```python
from build123d import *

# Parameters (mm, degrees)
SKETCH1_R           = 2.286
MAIN_BODY_DEPTH     = 1.5875
SKETCH2_R           = 2.286
MOUNT_HOLES_DEPTH   = 2.5875
SKETCH3_R           = 1.5875
OLD_PCB_HOLES_DEPTH = 2.54


with BuildPart() as part:
    # Sketch1 → Main Body (new body)
    with BuildSketch(Plane(origin=(0, 0, 0), x_dir=(1, 0, 0), z_dir=(0, 1, 0))):
        Polygon((-25.4, 86.995), (-63.43142, 86.995), (-63.43142, 60.96), (-78.74, 60.96), (-78.74, 25.4), (-71.12, 25.4), (-71.12, -25.4), (-78.74, -25.4), (-78.74, -60.96), (-63.43142, -60.96), (-63.43142, -86.995), (-25.4, -86.995), (-25.4, -79.375), (25.4, -79.375), (25.4, -86.995), (63.43142, -86.995), (63.43142, -60.96), (78.74, -60.96), (78.74, -25.4), (71.12, -25.4), (71.12, 25.4), (78.74, 25.4), (78.74, 60.96), (63.43142, 60.96), (63.43142, 86.995), (25.4, 86.995), (25.4, 79.375), (-25.4, 79.375), align=None)
        with Locations((-57.15, 76.2)):
            Circle(SKETCH1_R, mode=Mode.SUBTRACT)
        with Locations((57.15, 76.2)):
            Circle(SKETCH1_R, mode=Mode.SUBTRACT)
        with Locations((57.15, -76.2)):
            Circle(SKETCH1_R, mode=Mode.SUBTRACT)
        with Locations((-57.15, -76.2)):
            Circle(SKETCH1_R, mode=Mode.SUBTRACT)
    extrude(amount=MAIN_BODY_DEPTH)

    # Sketch2 → Mount Holes (cut, through all)
    with BuildSketch(Plane(origin=(0, 1.5875, 0), x_dir=(1, 0, 0), z_dir=(0, 1, 0))):
        with Locations((-73.66, -30.48)):
            Circle(SKETCH2_R)
        with Locations((-73.66, -55.88)):
            Circle(SKETCH2_R)
        with Locations((73.66, -55.88)):
            Circle(SKETCH2_R)
        with Locations((73.66, -30.48)):
            Circle(SKETCH2_R)
        with Locations((73.66, 30.48)):
            Circle(SKETCH2_R)
        with Locations((73.66, 55.88)):
            Circle(SKETCH2_R)
        with Locations((-73.66, 55.88)):
            Circle(SKETCH2_R)
        with Locations((-73.66, 30.48)):
            Circle(SKETCH2_R)
    extrude(amount=-MOUNT_HOLES_DEPTH, mode=Mode.SUBTRACT)

    # Sketch3 → Old PCB Holes (cut)
    with BuildSketch(Plane(origin=(0, 1.5875, 0), x_dir=(1, 0, 0), z_dir=(0, 1, 0))):
        with Locations((46.99, -59.69)):
            Circle(SKETCH3_R)
        with Locations((-46.99, -59.69)):
            Circle(SKETCH3_R)
        with Locations((-46.99, 59.69)):
            Circle(SKETCH3_R)
        with Locations((46.99, 59.69)):
            Circle(SKETCH3_R)
    extrude(amount=-OLD_PCB_HOLES_DEPTH, mode=Mode.SUBTRACT)


solid = part.part
```
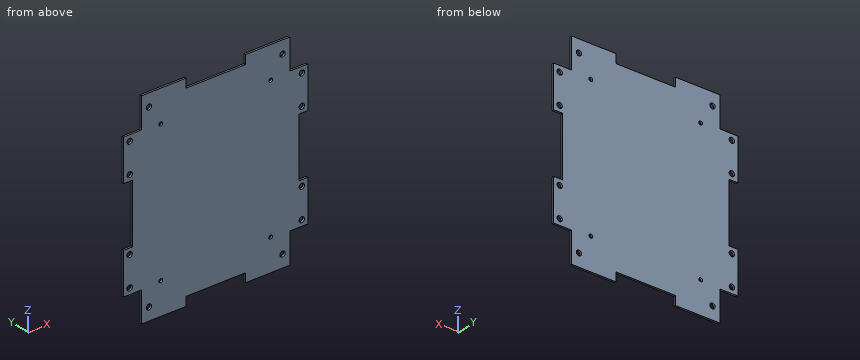
Part model, mm, in its own coordinate system. Round coordinates to 2 decimals unless told otherwise and drop trailing zeros. Loops run counter-clockwise (first coordinate to the right, second up) from the corner with the lowest first, then second, coordinate; pieces in that order, holes last. Notation, with made-up numbers: (-35.5, 27.25) -> (-3.5, 27.25) arc R24 cw to (-3.5, 63.25) -> close; hole circle Ø10 at (-32.5, 29.25). An arc over 180 degrees is marked (long way). Use CSV: the item, a comma, the result in double quotes. Start each with the question number.
1) Cut at A-A, the plane x = -73.66. Write the cut outline in (y, z).
2) Cut at C-C, the plane x = 57.15. Write the cut outline in (y, z) (1 decimal).
3) Cut at B-B, the plane z = 76.2. Write the cut outline in (x, y), plus the area to 3 significant figures.
4) Drop flat-ended pins along their axis: P1, Ø0.5, axis at x = -76, y = 0.5, coming from the +Z side; P2, Ø0.8, axis at x = 9, y = 0.5, coming from the +Z side (3 decimals); P3, Ø0.8, axis at y = 0.5, z = -82.5, coming from the -X side. Give the stop position or say it passes through.
5) Cut at D-D, the plane y = 1.2. Give the number of separate pieces and of enclosed holes in the cut face, plus the area to 3 significant figures.
6) Wall check: L1, parallel to X at y = 0.5, z = -30.48; L2, parallel to Z at x = 73.66, y = 0.8; L3, parallel to X at y = 0.8, z = -76.2. Give the ranges that are in metal, low to high. Write a range as [from, to].
Determined:
1,outline,"(0, -60.96) -> (1.59, -60.96) -> (1.59, -58.17) -> (0, -58.17) -> close; (0, -53.59) -> (1.59, -53.59) -> (1.59, -32.77) -> (0, -32.77) -> close; (0, -28.19) -> (1.59, -28.19) -> (1.59, -25.4) -> (0, -25.4) -> close; (0, 25.4) -> (1.59, 25.4) -> (1.59, 28.19) -> (0, 28.19) -> close; (0, 32.77) -> (1.59, 32.77) -> (1.59, 53.59) -> (0, 53.59) -> close; (0, 58.17) -> (1.59, 58.17) -> (1.59, 60.96) -> (0, 60.96) -> close"
2,outline,"(0, -87) -> (1.6, -87) -> (1.6, -78.5) -> (0, -78.5) -> close; (0, -73.9) -> (1.6, -73.9) -> (1.6, 73.9) -> (0, 73.9) -> close; (0, 78.5) -> (1.6, 78.5) -> (1.6, 87) -> (0, 87) -> close"
3,outline,"(-63.43, 0) -> (-59.44, 0) -> (-59.44, 1.59) -> (-63.43, 1.59) -> close; (-54.86, 0) -> (54.86, 0) -> (54.86, 1.59) -> (-54.86, 1.59) -> close; (59.44, 0) -> (63.43, 0) -> (63.43, 1.59) -> (59.44, 1.59) -> close"
3,area,"187 mm2"
4,P1,"stops at z = 60.96"
4,P2,"stops at z = 79.375"
4,P3,"stops at x = -63.43"
5,separate pieces,"1"
5,enclosed holes,"16"
5,area,"24,000 mm2"
6,L1,"x = [-78.74, -75.95], [-71.37, 71.37], [75.95, 78.74]"
6,L2,"z = [-60.96, -58.17], [-53.59, -32.77], [-28.19, -25.4], [25.4, 28.19], [32.77, 53.59], [58.17, 60.96]"
6,L3,"x = [-63.43, -59.44], [-54.86, 54.86], [59.44, 63.43]"
